Verification items for the finished model (mm, model axes). A direction names the side the tool comes from. Round coordinates to 2 decimals unless told otherwise and drop trailing zeros. Write each loop counter-clockwise with the first axis right and the second up, starting at its lowest first coordinate (ties: lowest second). Pieces come first, ordered by that corner, then holes. Notation, with made-up numbers: (88, 8.5) - (147, 8.5) arc R14 cw to (147, 19.5) - close; hole circle Ø1 at (-26.75, 18.5). An arc over 180 degrees is marked (long way). Answer as a JSON object with one key per item and string values.
```python
from build123d import *

# Parameters (mm, degrees)
SKETCH1_W            = 300
SKETCH1_H            = 20
BOSS_EXTRUDE1_DEPTH  = 8
SKETCH2_W            = 34
SKETCH2_H            = 8
BOSS_EXTRUDE2_DEPTH  = 9
SKETCH3_W            = 34
SKETCH3_H            = 8
BOSS_EXTRUDE3_DEPTH  = 9
SKETCH4_R            = 1.45
CUT_EXTRUDE1_DEPTH   = 302.504560496
SKETCH5_W            = 25
SKETCH5_H            = 8
BOSS_EXTRUDE4_DEPTH  = 17
SKETCH6_W            = 25
SKETCH6_H            = 8
BOSS_EXTRUDE5_DEPTH  = 17
SKETCH7_W            = 10
SKETCH7_H            = 38
CUT_EXTRUDE2_DEPTH   = 303.37890138
SKETCH8_W            = 7
SKETCH8_H            = 16
CUT_EXTRUDE3_DEPTH   = 4
CUT_EXTRUDE4_DEPTH   = 7
BOSS_EXTRUDE6_DEPTH  = 10
SKETCH12_W           = 8
SKETCH12_H           = 8
BOSS_EXTRUDE7_DEPTH  = 17
SKETCH13_R           = 1.7
CUT_EXTRUDE6_DEPTH   = 305.926220585
SKETCH14_W           = 20
SKETCH14_H           = 13
BOSS_EXTRUDE8_DEPTH  = 12
SKETCH15_R           = 1.6
CUT_EXTRUDE7_DEPTH   = 20
SKETCH16_W           = 20
SKETCH16_H           = 13
BOSS_EXTRUDE9_DEPTH  = 12
SKETCH17_R           = 1.6
CUT_EXTRUDE8_DEPTH   = 20
SKETCH18_W           = 20
SKETCH18_H           = 13
BOSS_EXTRUDE10_DEPTH = 12
CUT_EXTRUDE9_START   = -20
SKETCH19_R           = 1.6
CUT_EXTRUDE9_DEPTH   = 20
SKETCH20_W           = 20
SKETCH20_H           = 13
BOSS_EXTRUDE11_DEPTH = 12
CUT_EXTRUDE10_START  = -20
SKETCH21_R           = 1.6
CUT_EXTRUDE10_DEPTH  = 20
FILLET6_R            = 3
SKETCH28_W           = 198.881436238
SKETCH28_H           = 556.355103816
CUT_EXTRUDE14_DEPTH  = 220
SKETCH29_W           = 21
SKETCH29_H           = 8
BOSS_EXTRUDE12_DEPTH = 15
SKETCH30_W           = 21
SKETCH30_H           = 10
CUT_EXTRUDE15_DEPTH  = 306.0983448
SKETCH31_R           = 1.6
CUT_EXTRUDE16_DEPTH  = 306.0983448
FILLET7_R            = 3
SKETCH32_W           = 5.5
SKETCH32_H           = 70.463459777
CUT_EXTRUDE17_DEPTH  = 0.8
SKETCH33_W           = 20
SKETCH33_H           = 4.963841857
CUT_EXTRUDE18_DEPTH  = 0.5
SKETCH34_W           = 20
SKETCH34_H           = 11.942443484
CUT_EXTRUDE19_DEPTH  = 0.5


with BuildPart() as part:
    # Sketch1 → Boss-Extrude1 (new body)
    with BuildSketch(Plane(origin=(0, 0, 0), x_dir=(1, 0, 0), z_dir=(0, 1, 0))):
        with Locations((150, -10)):
            Rectangle(SKETCH1_W, SKETCH1_H)
    extrude(amount=BOSS_EXTRUDE1_DEPTH)

    # Sketch2 → Boss-Extrude2 (add)
    with BuildSketch(Plane.XY.offset(20)):
        with Locations((17, 4)):
            Rectangle(SKETCH2_W, SKETCH2_H)
        with Locations((283, 4)):
            Rectangle(SKETCH2_W, SKETCH2_H)
    extrude(amount=BOSS_EXTRUDE2_DEPTH)

    # Sketch3 → Boss-Extrude3 (add)
    with BuildSketch(Plane(origin=(0, 0, 0), x_dir=(-1, 0, 0), z_dir=(0, 0, -1))):
        with Locations((-17, 4)):
            Rectangle(SKETCH3_W, SKETCH3_H)
        with Locations((-283, 4)):
            Rectangle(SKETCH3_W, SKETCH3_H)
    extrude(amount=BOSS_EXTRUDE3_DEPTH)

    # Sketch4 → Cut-Extrude1 (cut, through all)
    with BuildSketch(Plane(origin=(0, 8, 0), x_dir=(1, 0, 0), z_dir=(0, 1, 0))):
        with Locations(Location((4, 5, 0), (0, 0, 270))):
            Circle(SKETCH4_R)
        with Locations(Location((30, 5, 0), (0, 0, 270))):
            Circle(SKETCH4_R)
        with Locations(Location((30, -25, 0), (0, 0, 270))):
            Circle(SKETCH4_R)
        with Locations(Location((4, -25, 0), (0, 0, 270))):
            Circle(SKETCH4_R)
        with Locations(Location((296, -25, 0), (0, 0, 270))):
            Circle(SKETCH4_R)
        with Locations(Location((296, 5, 0), (0, 0, 270))):
            Circle(SKETCH4_R)
        with Locations(Location((270, -25, 0), (0, 0, 270))):
            Circle(SKETCH4_R)
        with Locations(Location((270, 5, 0), (0, 0, 270))):
            Circle(SKETCH4_R)
    extrude(amount=-CUT_EXTRUDE1_DEPTH, mode=Mode.SUBTRACT)

    # Sketch5 → Boss-Extrude4 (add)
    with BuildSketch(Plane.XY.offset(20)):
        with Locations((253.5, 4)):
            Rectangle(SKETCH5_W, SKETCH5_H)
    extrude(amount=BOSS_EXTRUDE4_DEPTH)

    # Sketch6 → Boss-Extrude5 (add)
    with BuildSketch(Plane(origin=(0, 0, 0), x_dir=(-1, 0, 0), z_dir=(0, 0, -1))):
        with Locations((-253.5, 4)):
            Rectangle(SKETCH6_W, SKETCH6_H)
    extrude(amount=BOSS_EXTRUDE5_DEPTH)

    # Sketch7 → Cut-Extrude2 (cut, through all)
    with BuildSketch(Plane(origin=(0, 8, 0), x_dir=(1, 0, 0), z_dir=(0, 1, 0))):
        with Locations((254, -10)):
            Rectangle(SKETCH7_W, SKETCH7_H)
    extrude(amount=-CUT_EXTRUDE2_DEPTH, mode=Mode.SUBTRACT)

    # Sketch8 → Cut-Extrude3 (cut)
    with BuildSketch(Plane(origin=(0, 8, 0), x_dir=(1, 0, 0), z_dir=(0, 1, 0))):
        with Locations((262.5, -10)):
            Rectangle(SKETCH8_W, SKETCH8_H)
    extrude(amount=-CUT_EXTRUDE3_DEPTH, mode=Mode.SUBTRACT)

    # Sketch9 → Cut-Extrude4 (cut)
    with BuildSketch(Plane.ZY.offset(-259)):
        Polygon((18, 4), (22, 8), (18, 8), align=None)
        Polygon((2, 4), (-2, 8), (2, 8), align=None)
    extrude(amount=-CUT_EXTRUDE4_DEPTH, mode=Mode.SUBTRACT)

    # Sketch10 → Boss-Extrude6 (add)
    with BuildSketch(Plane.ZY.offset(-259)):
        Polygon((-2, 0), (-9, 8), (-9, 0), align=None)
        Polygon((29, 8), (22, 0), (29, 0), align=None)
    extrude(amount=BOSS_EXTRUDE6_DEPTH)

    # Sketch12 → Boss-Extrude7 (add)
    with BuildSketch(Plane.XY.offset(37)):
        with Locations((245, 4)):
            Rectangle(SKETCH12_W, SKETCH12_H)
    extrude(amount=BOSS_EXTRUDE7_DEPTH)

    # Sketch13 → Cut-Extrude6 (cut, through all)
    with BuildSketch(Plane(origin=(0, 8, 0), x_dir=(1, 0, 0), z_dir=(0, 1, 0))):
        with Locations(Location((245, -50, 0), (0, 0, 270))):
            Circle(SKETCH13_R)
        with Locations(Location((245, -18, 0), (0, 0, 270))):
            Circle(SKETCH13_R)
    extrude(amount=-CUT_EXTRUDE6_DEPTH, mode=Mode.SUBTRACT)

    # Sketch14 → Boss-Extrude8 (add)
    with BuildSketch(Plane.XY.offset(29)):
        with Locations((285, 6.5)):
            Rectangle(SKETCH14_W, SKETCH14_H)
    extrude(amount=BOSS_EXTRUDE8_DEPTH)

    # Sketch15 → Cut-Extrude7 (cut)
    with BuildSketch(Plane(origin=(295, 0, 0), x_dir=(0, 0, -1), z_dir=(1, 0, 0))):
        with Locations((-35, 8)):
            Circle(SKETCH15_R)
    extrude(amount=-CUT_EXTRUDE7_DEPTH, mode=Mode.SUBTRACT)

    # Sketch16 → Boss-Extrude9 (add)
    with BuildSketch(Plane(origin=(0, 0, -9), x_dir=(-1, 0, 0), z_dir=(0, 0, -1))):
        with Locations((-285, 6.5)):
            Rectangle(SKETCH16_W, SKETCH16_H)
    extrude(amount=BOSS_EXTRUDE9_DEPTH)

    # Sketch17 → Cut-Extrude8 (cut)
    with BuildSketch(Plane(origin=(295, 0, 0), x_dir=(0, 0, -1), z_dir=(1, 0, 0))):
        with Locations((15, 8)):
            Circle(SKETCH17_R)
    extrude(amount=-CUT_EXTRUDE8_DEPTH, mode=Mode.SUBTRACT)

    # Sketch18 → Boss-Extrude10 (add)
    with BuildSketch(Plane(origin=(0, 0, -9), x_dir=(-1, 0, 0), z_dir=(0, 0, -1))):
        with Locations((-15, 6.5)):
            Rectangle(SKETCH18_W, SKETCH18_H)
    extrude(amount=BOSS_EXTRUDE10_DEPTH)

    # Sketch19 → Cut-Extrude9 (cut)
    with BuildSketch(Plane.ZY.offset(-5).offset(CUT_EXTRUDE9_START)):
        with Locations(Location((-15, 8, 0), (0, 0, 180))):
            Circle(SKETCH19_R)
    extrude(amount=CUT_EXTRUDE9_DEPTH, mode=Mode.SUBTRACT)

    # Sketch20 → Boss-Extrude11 (add)
    with BuildSketch(Plane.XY.offset(29)):
        with Locations((15, 6.5)):
            Rectangle(SKETCH20_W, SKETCH20_H)
    extrude(amount=BOSS_EXTRUDE11_DEPTH)

    # Sketch21 → Cut-Extrude10 (cut)
    with BuildSketch(Plane.ZY.offset(-5).offset(CUT_EXTRUDE10_START)):
        with Locations(Location((35, 8, 0), (0, 0, 180))):
            Circle(SKETCH21_R)
    extrude(amount=CUT_EXTRUDE10_DEPTH, mode=Mode.SUBTRACT)

    # Fillet6
    fillet6_edges = [part.edges().sort_by_distance(p)[0] for p in [
        (285, 13, 29),
        (285, 13, 41),
        (285, 13, -9),
        (285, 13, -21),
        (15, 13, -9),
        (15, 13, -21),
        (15, 13, 29),
        (15, 13, 41),
    ]]
    fillet(fillet6_edges, radius=FILLET6_R)

    # Sketch28 → Cut-Extrude14 (cut)
    with BuildSketch(Plane.ZY):
        with Locations((-20.495432896, -60.484201615)):
            Rectangle(SKETCH28_W, SKETCH28_H)
    extrude(amount=-CUT_EXTRUDE14_DEPTH, mode=Mode.SUBTRACT)

    # Sketch29 → Boss-Extrude12 (add)
    with BuildSketch(Plane(origin=(0, 0, 0), x_dir=(-1, 0, 0), z_dir=(0, 0, -1))):
        with Locations((-230.5, 4)):
            Rectangle(SKETCH29_W, SKETCH29_H)
    extrude(amount=BOSS_EXTRUDE12_DEPTH)

    # Sketch30 → Cut-Extrude15 (cut, through all)
    with BuildSketch(Plane(origin=(0, 0, 0), x_dir=(-1, 0, 0), z_dir=(0, -1, 0))):
        with Locations((-230.5, -15)):
            Rectangle(SKETCH30_W, SKETCH30_H)
    extrude(amount=-CUT_EXTRUDE15_DEPTH, mode=Mode.SUBTRACT)

    # Sketch31 → Cut-Extrude16 (cut, through all)
    with BuildSketch(Plane(origin=(0, 0, 0), x_dir=(-1, 0, 0), z_dir=(0, -1, 0))):
        with Locations(Location((-225, 7, 0), (0, 0, 90))):
            Circle(SKETCH31_R)
        with Locations(Location((-225, -3, 0), (0, 0, 90))):
            Circle(SKETCH31_R)
        with Locations(Location((-233, 7, 0), (0, 0, 90))):
            Circle(SKETCH31_R)
        with Locations(Location((-233, -3, 0), (0, 0, 90))):
            Circle(SKETCH31_R)
    extrude(amount=-CUT_EXTRUDE16_DEPTH, mode=Mode.SUBTRACT)

    # Fillet7
    fillet7_edges = [part.edges().sort_by_distance(p)[0] for p in [
        (300, 4, 29),
        (300, 4, -9),
    ]]
    fillet(fillet7_edges, radius=FILLET7_R)

    # Sketch32 → Cut-Extrude17 (cut)
    with BuildSketch(Plane(origin=(0, 13, 0), x_dir=(1, 0, 0), z_dir=(0, 1, 0))):
        with Locations((285, -7.2213573)):
            Rectangle(SKETCH32_W, SKETCH32_H)
    extrude(amount=-CUT_EXTRUDE17_DEPTH, mode=Mode.SUBTRACT)

    # Sketch33 → Cut-Extrude18 (cut)
    with BuildSketch(Plane(origin=(0, 0, 29), x_dir=(-1, 0, 0), z_dir=(0, 0, -1))):
        with Locations((-285, 10.481920928)):
            Rectangle(SKETCH33_W, SKETCH33_H)
    extrude(amount=-CUT_EXTRUDE18_DEPTH, mode=Mode.SUBTRACT)

    # Sketch34 → Cut-Extrude19 (cut)
    with BuildSketch(Plane.XY.offset(-9)):
        with Locations((285, 13.971221742)):
            Rectangle(SKETCH34_W, SKETCH34_H)
    extrude(amount=-CUT_EXTRUDE19_DEPTH, mode=Mode.SUBTRACT)


solid = part.part
```
Q1. Set-up check for faces 3 (the flat face through (231, 4, 10)), 4 (the flat face through (271, 4, -9)), 5 (the flat face through (254, 4, -17)), 6 (the flat face through (259, 3, 10)), 7 (the flat face through (269, 8, 11)): record each of +Z, -Z, +X, -X, +Y, -Y from which the full face is reachable in a straight line by a thin tool's end or side.
Geometry check:
{"face 3": "+Z, -X, +Y, -Y", "face 4": "-Z, +Y, -Y", "face 5": "-Z, -X, +Y, -Y", "face 6": "+Y", "face 7": "-X, +Y"}
Q2. Section check A-A, the plane z = 8. Record the cut outline in (x, y), then the cut area to 3 significant figures.
Geometry check:
{"outline": "(220, 0) - (249, 0) - (249, 8) - (220, 8) - close; (259, 0) - (300, 0) - (300, 8) - (266, 8) - (266, 4) - (259, 4) - close", "area": "532 mm2"}
Q3. Section check D-D, the plane z = 50. Record the cut outline in (x, y), then the cut area to 3 significant figures.
Geometry check:
{"outline": "(241, 0) - (243.3, 0) - (243.3, 8) - (241, 8) - close; (246.7, 0) - (249, 0) - (249, 8) - (246.7, 8) - close", "area": "36.8 mm2"}
Q4. Gauge pin test, flat ends, axial feed: P1, Ø6.5, axis at y = 2.5, z = 33, coming from the +X side; P2, Ø4, axis at x = 270, z = -5, coming from the -Y side; P3, Ø6.5, axis at y = 2, z = 15, coming from the -X side; P4, Ø5, axis at x = 233, z = -7, coming from the +Y side. Record the tip position at first contact, or that the pin passes through.
Geometry check:
{"P1": "stops at x = 295", "P2": "stops at y = 0", "P3": "stops at x = 241", "P4": "stops at y = 8"}
Q5. Section check B-B, the plane x = 245. Record the cut outline in (y, z).
Geometry check:
{"outline": "(0, -17) - (8, -17) - (8, 16.3) - (0, 16.3) - close; (0, 19.7) - (8, 19.7) - (8, 48.3) - (0, 48.3) - close; (0, 51.7) - (8, 51.7) - (8, 54) - (0, 54) - close"}
Q6. Release check for a two-part mould opening along X. For faces 1 (the flat face through (285, 5, -21)), 2 (the flat face through (262, 4, 10)) record: released by +X, released by -X, zero draft, split by the parting line, or undercut.
Geometry check:
{"face 1": "zero draft", "face 2": "undercut"}
Q7. Material ranges on line 1 along X through (y, z) = (6, -5); line 2 along Z through (x, y) = (225, 4.5); line 3 along Z through (x, y) = (270, 5), recorded low to high. Write a range as [from, to].
Geometry check:
{"line 1": "x = [220, 249], [259, 268.55], [271.45, 294.55], [297.45, 300]", "line 2": "z = [-15, -8.6], [-5.4, 1.4], [4.6, 10]", "line 3": "z = [-9, -6.45], [-3.55, 23.55], [26.45, 29]"}
Q8. Section check C-C, the plane z = 25. Record the cut outline in (x, y).
Geometry check:
{"outline": "(241, 0) - (268.55, 0) - (268.55, 8) - (259, 8) - (259, 3.43) - (249, 3.43) - (249, 8) - (241, 8) - close; (271.45, 0) - (294.55, 0) - (294.55, 8) - (271.45, 8) - close; (297.45, 0) - (300, 0) - (300, 8) - (297.45, 8) - close"}
